from build123d import *

# Parameters (mm, degrees)
F_01_HOUSING_DEPTH        = 62
SKETCH_2_W                = 50
SKETCH_2_H                = 24
F_02_COLUMN_DEPTH         = 62
F_03_BASE_DEPTH           = 12
SKETCH_4_R                = 32
F_04_SBOX_DEPTH           = 35
SKETCH_5_R                = 24
F_05_CAV_UP_DEPTH         = 30
SKETCH_6_R                = 9
F_06_BRG_UP_DEPTH         = 20
SKETCH_7_R                = 13
F_07_PACK_UP_DEPTH        = 22
SKETCH_8_R                = 17.25
F_08_M36_UP_DEPTH         = 25
SKETCH_9_R                = 24
F_09_CAV_LO_DEPTH         = 30
SKETCH_10_R               = 9
F_10_BRG_LO_DEPTH         = 20
SKETCH_11_R               = 15
F_11_RECESS_LO_DEPTH      = 12
SKETCH_12_R               = 15
F_12_PORTBOSS_P_DEPTH     = 17
SKETCH_13_R               = 10
F_13_PASS_P_DEPTH         = 25
SKETCH_14_R               = 5.9
F_14_G14_P_DEPTH          = 14
F_12_PORTBOSS_N_START     = -17
SKETCH_15_R               = 15
F_12_PORTBOSS_N_DEPTH     = 17
F_13_PASS_N_START         = 25
SKETCH_16_R               = 10
F_13_PASS_N_DEPTH         = 25
F_14_G14_N_START          = 14
SKETCH_17_R               = 5.9
F_14_G14_N_DEPTH          = 14
SKETCH_18_R               = 2.5
CUT_EXTRUDE_15_M6_0_DEPTH = 10
SKETCH_19_R               = 2.5
CUT_EXTRUDE_15_M6_1_DEPTH = 10
SKETCH_20_R               = 2.5
CUT_EXTRUDE_15_M6_2_DEPTH = 10
SKETCH_21_R               = 2.5
CUT_EXTRUDE_15_M6_3_DEPTH = 10
SKETCH_22_R               = 2.5
CUT_EXTRUDE_15_M6_4_DEPTH = 10
SKETCH_23_R               = 2.5
CUT_EXTRUDE_15_M6_5_DEPTH = 10
SKETCH_24_R               = 2.5
F_16_DOWEL_0_DEPTH        = 12
SKETCH_25_R               = 2.5
F_16_DOWEL_1_DEPTH        = 12
SKETCH_26_R               = 4.5
F_17_BH_00_DEPTH          = 14
SKETCH_27_R               = 4.5
F_17_BH_01_DEPTH          = 14
SKETCH_28_R               = 4.5
F_17_BH_10_DEPTH          = 14
SKETCH_29_R               = 4.5
F_17_BH_11_DEPTH          = 14
SKETCH_30_R               = 4.5
F_17_BH_20_DEPTH          = 14
SKETCH_31_R               = 4.5
F_17_BH_21_DEPTH          = 14
SKETCH_32_R               = 4.5
F_17_BH_30_DEPTH          = 14
SKETCH_33_R               = 4.5
F_17_BH_31_DEPTH          = 14
SKETCH_34_W               = 78
SKETCH_34_H               = 42
F_18_RELIEF_DEPTH         = 4


with BuildPart() as part:
    # Sketch 1 → 01_HOUSING (new body)
    with BuildSketch(Plane(origin=(-30, 0, 0), x_dir=(0, 0, -1), z_dir=(1, 0, 0))):
        with BuildLine():
            Line((-104, -40), (-62, -40))
            ThreePointArc((-62, -40), (-22, 0), (-62, 40))
            Line((-62, 40), (-104, 40))
            ThreePointArc((-104, 40), (-144, 0), (-104, -40))
        make_face()
    extrude(amount=F_01_HOUSING_DEPTH)

    # Sketch 2 → 02_COLUMN (add)
    with BuildSketch(Plane(origin=(-30, 0, 0), x_dir=(0, 0, -1), z_dir=(1, 0, 0))):
        with Locations((-37, 0)):
            Rectangle(SKETCH_2_W, SKETCH_2_H)
    extrude(amount=F_02_COLUMN_DEPTH)

    # Sketch 3 → 03_BASE (add)
    with BuildSketch(Plane.XY):
        Polygon((26, -44), (27.552914271, -43.795554958), (29, -43.196152423), (30.242640687, -42.242640687), (31.196152423, -41), (31.795554958, -39.552914271), (32, -38), (32, 38), (31.795554958, 39.552914271), (31.196152423, 41), (30.242640687, 42.242640687), (29, 43.196152423), (27.552914271, 43.795554958), (26, 44), (-40, 44), (-41.552914271, 43.795554958), (-43, 43.196152423), (-44.242640687, 42.242640687), (-45.196152423, 41), (-45.795554958, 39.552914271), (-46, 38), (-46, -38), (-45.795554958, -39.552914271), (-45.196152423, -41), (-44.242640687, -42.242640687), (-43, -43.196152423), (-41.552914271, -43.795554958), (-40, -44), align=None)
    extrude(amount=F_03_BASE_DEPTH)

    # Sketch 4 → 04_SBOX (add)
    with BuildSketch(Plane(origin=(32, 0, 0), x_dir=(0, 0, -1), z_dir=(1, 0, 0))):
        with Locations((-104, 0)):
            Circle(SKETCH_4_R)
    extrude(amount=F_04_SBOX_DEPTH)

    # Sketch 5 → 05_CAV_UP (cut)
    with BuildSketch(Plane(origin=(-30, 0, 0), x_dir=(0, 0, -1), z_dir=(1, 0, 0))):
        with Locations((-104, 0)):
            Circle(SKETCH_5_R)
    extrude(amount=F_05_CAV_UP_DEPTH, mode=Mode.SUBTRACT)

    # Sketch 6 → 06_BRG_UP (cut)
    with BuildSketch(Plane(origin=(0, 0, 0), x_dir=(0, 0, -1), z_dir=(1, 0, 0))):
        with Locations((-104, 0)):
            Circle(SKETCH_6_R)
    extrude(amount=F_06_BRG_UP_DEPTH, mode=Mode.SUBTRACT)

    # Sketch 7 → 07_PACK_UP (cut)
    with BuildSketch(Plane(origin=(20, 0, 0), x_dir=(0, 0, -1), z_dir=(1, 0, 0))):
        with Locations((-104, 0)):
            Circle(SKETCH_7_R)
    extrude(amount=F_07_PACK_UP_DEPTH, mode=Mode.SUBTRACT)

    # Sketch 8 → 08_M36_UP (cut)
    with BuildSketch(Plane(origin=(42, 0, 0), x_dir=(0, 0, -1), z_dir=(1, 0, 0))):
        with Locations((-104, 0)):
            Circle(SKETCH_8_R)
    extrude(amount=F_08_M36_UP_DEPTH, mode=Mode.SUBTRACT)

    # Sketch 9 → 09_CAV_LO (cut)
    with BuildSketch(Plane(origin=(-30, 0, 0), x_dir=(0, 0, -1), z_dir=(1, 0, 0))):
        with Locations((-62, 0)):
            Circle(SKETCH_9_R)
    extrude(amount=F_09_CAV_LO_DEPTH, mode=Mode.SUBTRACT)

    # Sketch 10 → 10_BRG_LO (cut)
    with BuildSketch(Plane(origin=(0, 0, 0), x_dir=(0, 0, -1), z_dir=(1, 0, 0))):
        with Locations((-62, 0)):
            Circle(SKETCH_10_R)
    extrude(amount=F_10_BRG_LO_DEPTH, mode=Mode.SUBTRACT)

    # Sketch 11 → 11_RECESS_LO (cut)
    with BuildSketch(Plane(origin=(20, 0, 0), x_dir=(0, 0, -1), z_dir=(1, 0, 0))):
        with Locations(Location((-62, 0, 0), (0, 0, 220.015277982))):
            Circle(SKETCH_11_R)
    extrude(amount=F_11_RECESS_LO_DEPTH, mode=Mode.SUBTRACT)

    # Sketch 12 → 12_PORTBOSS_P (add)
    with BuildSketch(Plane(origin=(0, 30, 0), x_dir=(1, 0, 0), z_dir=(0, 1, 0))):
        with Locations(Location((-14, -83, 0), (0, 0, 90))):
            Circle(SKETCH_12_R)
    extrude(amount=F_12_PORTBOSS_P_DEPTH)

    # Sketch 13 → 13_PASS_P (cut)
    with BuildSketch(Plane(origin=(0, 33, 0), x_dir=(1, 0, 0), z_dir=(0, 1, 0))):
        with Locations(Location((-14, -83, 0), (0, 0, 270))):
            Circle(SKETCH_13_R)
    extrude(amount=-F_13_PASS_P_DEPTH, mode=Mode.SUBTRACT)

    # Sketch 14 → 14_G14_P (cut)
    with BuildSketch(Plane(origin=(0, 47, 0), x_dir=(1, 0, 0), z_dir=(0, 1, 0))):
        with Locations(Location((-14, -83, 0), (0, 0, 270))):
            Circle(SKETCH_14_R)
    extrude(amount=-F_14_G14_P_DEPTH, mode=Mode.SUBTRACT)

    # Sketch 15 → 12_PORTBOSS_N (add)
    with BuildSketch(Plane(origin=(0, -30, 0), x_dir=(1, 0, 0), z_dir=(0, 1, 0)).offset(F_12_PORTBOSS_N_START)):
        with Locations(Location((-14, -83, 0), (0, 0, 90))):
            Circle(SKETCH_15_R)
    extrude(amount=F_12_PORTBOSS_N_DEPTH)

    # Sketch 16 → 13_PASS_N (cut)
    with BuildSketch(Plane(origin=(0, -33, 0), x_dir=(1, 0, 0), z_dir=(0, 1, 0)).offset(F_13_PASS_N_START)):
        with Locations(Location((-14, -83, 0), (0, 0, 270))):
            Circle(SKETCH_16_R)
    extrude(amount=-F_13_PASS_N_DEPTH, mode=Mode.SUBTRACT)

    # Sketch 17 → 14_G14_N (cut)
    with BuildSketch(Plane(origin=(0, -47, 0), x_dir=(1, 0, 0), z_dir=(0, 1, 0)).offset(F_14_G14_N_START)):
        with Locations(Location((-14, -83, 0), (0, 0, 270))):
            Circle(SKETCH_17_R)
    extrude(amount=-F_14_G14_N_DEPTH, mode=Mode.SUBTRACT)

    # Sketch 18 → Cut-Extrude 15_M6_0 (cut)
    with BuildSketch(Plane(origin=(-30, 0, 0), x_dir=(0, 0, -1), z_dir=(1, 0, 0))):
        with Locations((-104, 32)):
            Circle(SKETCH_18_R)
    extrude(amount=CUT_EXTRUDE_15_M6_0_DEPTH, mode=Mode.SUBTRACT)

    # Sketch 19 → Cut-Extrude 15_M6_1 (cut)
    with BuildSketch(Plane(origin=(-30, 0, 0), x_dir=(0, 0, -1), z_dir=(1, 0, 0))):
        with Locations((-104, -32)):
            Circle(SKETCH_19_R)
    extrude(amount=CUT_EXTRUDE_15_M6_1_DEPTH, mode=Mode.SUBTRACT)

    # Sketch 20 → Cut-Extrude 15_M6_2 (cut)
    with BuildSketch(Plane(origin=(-30, 0, 0), x_dir=(0, 0, -1), z_dir=(1, 0, 0))):
        with Locations((-62, 32)):
            Circle(SKETCH_20_R)
    extrude(amount=CUT_EXTRUDE_15_M6_2_DEPTH, mode=Mode.SUBTRACT)

    # Sketch 21 → Cut-Extrude 15_M6_3 (cut)
    with BuildSketch(Plane(origin=(-30, 0, 0), x_dir=(0, 0, -1), z_dir=(1, 0, 0))):
        with Locations((-62, -32)):
            Circle(SKETCH_21_R)
    extrude(amount=CUT_EXTRUDE_15_M6_3_DEPTH, mode=Mode.SUBTRACT)

    # Sketch 22 → Cut-Extrude 15_M6_4 (cut)
    with BuildSketch(Plane(origin=(-30, 0, 0), x_dir=(0, 0, -1), z_dir=(1, 0, 0))):
        with Locations((-136, 0)):
            Circle(SKETCH_22_R)
    extrude(amount=CUT_EXTRUDE_15_M6_4_DEPTH, mode=Mode.SUBTRACT)

    # Sketch 23 → Cut-Extrude 15_M6_5 (cut)
    with BuildSketch(Plane(origin=(-30, 0, 0), x_dir=(0, 0, -1), z_dir=(1, 0, 0))):
        with Locations((-30, 0)):
            Circle(SKETCH_23_R)
    extrude(amount=CUT_EXTRUDE_15_M6_5_DEPTH, mode=Mode.SUBTRACT)

    # Sketch 24 → 16_DOWEL_0 (cut)
    with BuildSketch(Plane(origin=(-30, 0, 0), x_dir=(0, 0, -1), z_dir=(1, 0, 0))):
        with Locations((-126.6, 22.6)):
            Circle(SKETCH_24_R)
    extrude(amount=F_16_DOWEL_0_DEPTH, mode=Mode.SUBTRACT)

    # Sketch 25 → 16_DOWEL_1 (cut)
    with BuildSketch(Plane(origin=(-30, 0, 0), x_dir=(0, 0, -1), z_dir=(1, 0, 0))):
        with Locations((-39.4, -22.6)):
            Circle(SKETCH_25_R)
    extrude(amount=F_16_DOWEL_1_DEPTH, mode=Mode.SUBTRACT)

    # Sketch 26 → 17_BH_00 (cut)
    with BuildSketch(Plane.XY.offset(-1)):
        with Locations((-38, 40)):
            Circle(SKETCH_26_R)
    extrude(amount=F_17_BH_00_DEPTH, mode=Mode.SUBTRACT)

    # Sketch 27 → 17_BH_01 (cut)
    with BuildSketch(Plane.XY.offset(-1)):
        with Locations((-38, -40)):
            Circle(SKETCH_27_R)
    extrude(amount=F_17_BH_01_DEPTH, mode=Mode.SUBTRACT)

    # Sketch 28 → 17_BH_10 (cut)
    with BuildSketch(Plane.XY.offset(-1)):
        with Locations((-18, 40)):
            Circle(SKETCH_28_R)
    extrude(amount=F_17_BH_10_DEPTH, mode=Mode.SUBTRACT)

    # Sketch 29 → 17_BH_11 (cut)
    with BuildSketch(Plane.XY.offset(-1)):
        with Locations((-18, -40)):
            Circle(SKETCH_29_R)
    extrude(amount=F_17_BH_11_DEPTH, mode=Mode.SUBTRACT)

    # Sketch 30 → 17_BH_20 (cut)
    with BuildSketch(Plane.XY.offset(-1)):
        with Locations((4, 40)):
            Circle(SKETCH_30_R)
    extrude(amount=F_17_BH_20_DEPTH, mode=Mode.SUBTRACT)

    # Sketch 31 → 17_BH_21 (cut)
    with BuildSketch(Plane.XY.offset(-1)):
        with Locations((4, -40)):
            Circle(SKETCH_31_R)
    extrude(amount=F_17_BH_21_DEPTH, mode=Mode.SUBTRACT)

    # Sketch 32 → 17_BH_30 (cut)
    with BuildSketch(Plane.XY.offset(-1)):
        with Locations((24, 40)):
            Circle(SKETCH_32_R)
    extrude(amount=F_17_BH_30_DEPTH, mode=Mode.SUBTRACT)

    # Sketch 33 → 17_BH_31 (cut)
    with BuildSketch(Plane.XY.offset(-1)):
        with Locations((24, -40)):
            Circle(SKETCH_33_R)
    extrude(amount=F_17_BH_31_DEPTH, mode=Mode.SUBTRACT)

    # Sketch 34 → 18_RELIEF (cut)
    with BuildSketch(Plane.XY.offset(-1)):
        with Locations((-7, 0)):
            Rectangle(SKETCH_34_W, SKETCH_34_H)
    extrude(amount=F_18_RELIEF_DEPTH, mode=Mode.SUBTRACT)


solid = part.part
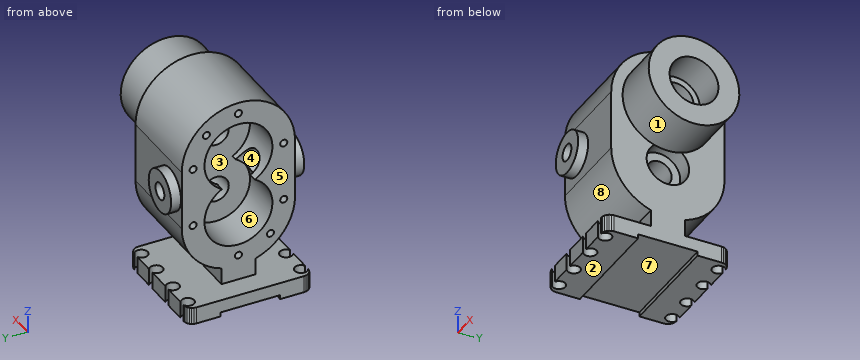
Part model, mm, in its own coordinate system. Face numbers are marked on the shaded views. A direction names the side the tool comes from. Coordinates: 2 decimals unless noted, no trailing zeros. Write each loop counter-clockwise with the first axis right and the second up, starting at its lowest first coordinate (ties: lowest second). Pieces come first, ordered by that corner, then holes. Notation, with made-up numbers: M 37.5,59 L 49.5,59 A15 cw 49.5,70 Z; hole C -4,71.5 d11. An arc over 180 degrees is marked long. Return JSON: item names as keys, results as strings.
1. Probe L1, parallel to Y at x = -21, z = 62; L2, parallel to X at y = -40, z = 9; L3, parallel to X at y = 13.5, z = 27. List the from-to ranges inside material, lowest first.
Determined:
{"L1": "-40 to -34.5, -29.5 to -24, 24 to 29.5, 34.5 to 40", "L2": "-45.61 to -42.5, -33.5 to -22.5, -13.5 to -0.5, 8.5 to 19.5, 28.5 to 31.61", "L3": "-30 to 32"}
2. Pull direction Y, two halves, no side cores. Call the marked faces 1, 2, 3 and 4: pulls with the +Y half, pulls with the -Y half, needs draft (parallel to the pull), parting line crosses it, or undercut.
Determined:
{"face 1": "parting line crosses it", "face 2": "needs draft", "face 3": "undercut", "face 4": "undercut"}
3. Flat gauge pins, fed straight in: pin 1 Ø10 at (x, y) = (18, 16) entering from +Z; pin 2 Ø8 at (y, z) = (-33, 81.5) entering from -X; pin 3 Ø9.5 at (x, z) = (-4.5, 4.5) entering from -Y. Where does each tip first touch, or does it go through?
Determined:
{"pin 1": "z = 142.46", "pin 2": "x = -30", "pin 3": "y = -44"}
4. Saw through at B-B, the plane y = 0. Count the separate pieces of the cut face and the enclosed holes in it, then the cut area to 3 significant figures.
Determined:
{"separate pieces": "3", "enclosed holes": "0", "area": "5,810 mm²"}
5. Saw through at A-A, the plane x = 11. Write the cut outline in (y, z).
Determined:
{"outline": "M -44,0 L -21,0 L -21,3 L 21,3 L 21,0 L 44,0 L 44,12 L 12,12 L 12,23.84 A40 ccw 40,62 L 40,104 A40 ccw -40,104 L -40,62 A40 ccw -12,23.84 L -12,12 L -44,12 Z; hole C 0,62 d18; hole C 0,104 d18"}
6. Saw through at D-D, the plane x = 54. Write the cut outline in (y, z), then the cut area to 3 significant figures.
Determined:
{"outline": "C 0,104 d64; hole C 0,104 d34.5", "area": "2,280 mm²"}
7. 3-axis set-ups, long thin cutter, end or side, ignore diameter. For the marked faces 5, 6, 7 and 8: which of +Z, -Z, +X, -X, +Y, -Y reach the whole face in a straight line?
Determined:
{"face 5": "+Z, -X, +Y, -Y", "face 6": "-X", "face 7": "-Z, +X, -X", "face 8": "+X, -X, -Y"}
